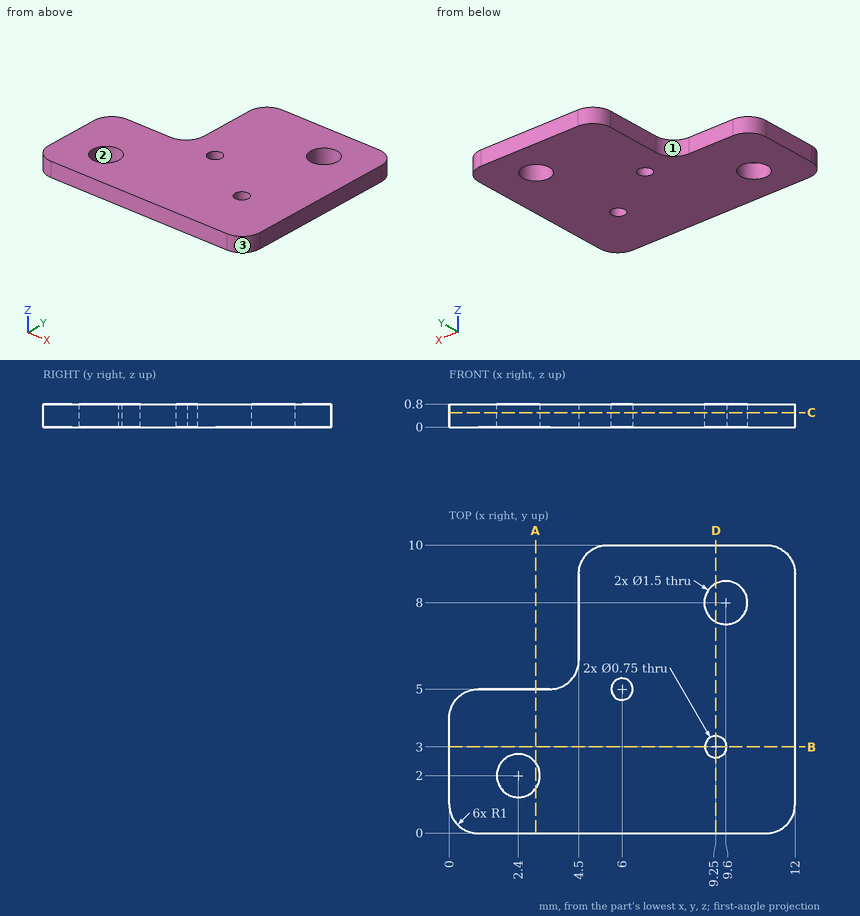
Geometry: see drawing. Coordinates: mm, zero at the bounding-box minimum. Round coordinates to 2 decimals unless told otherwise and drop trailing zeros. Loops run counter-clockwise (first coordinate to the right, second up) from the corner with the lowest first, then second, coordinate; pieces in that order, holes last. Notation, with made-up numbers: M 86.5,16 L 106.5,16 A33 ccw 106.5,55 Z; hole C 15.5,5 d8. An arc over 180 degrees is marked long. Use a Markdown table: item, result. Add a question column.
1. Contact query for a flat-ended pin moving along its axis: pin 1 (1.2 mm diameter, centred on x = 2.4, y = 2, fed in from -Z). Output: stop coordinate, or through.
2. Cut plane D-D, the plane x = 9.25. Output: boundary loops of the cut face in (y, z) (3 decimals).
3. Cut plane A-A, the plane x = 3. Output: boundary loops of the cut face in (y, z), and give its area (3 significant figures).
4. Pull-direction query (Y, two-part tool) for the marked faces 1, 2 and 3; classes: +Y half, -Y half, draft (parallel to the pull), parting line (faces both ways), or undercut.
5. Cut plane C-C, the plane z = 0.5. Output: boundary loops of the cut face in (x, y) (3 decimals), and give its area (3 significant figures).
6. Cut plane B-B, the plane y = 3. Output: boundary loops of the cut face in (x, z) (3 decimals).
7. Ray query, line 1 along Y through (x, z) = (9.25, 0.55) (3 decimals); line 2 along Y through (x, z) = (6, 0.45) (3 decimals); line 3 along X through (y, z) = (9, 0.1). Return the intervals inside material, ascending. Write a range as [from, to].
Solution:
| question | item | result |
|---|---|---|
| 1 | pin 1 | passes through |
| 2 | outline | M 0,0 L 2.625,0 L 2.625,0.8 L 0,0.8 Z; M 3.375,0 L 7.337,0 L 7.337,0.8 L 3.375,0.8 Z; M 8.663,0 L 10,0 L 10,0.8 L 8.663,0.8 Z |
| 3 | outline | M 0,0 L 1.55,0 L 1.55,0.8 L 0,0.8 Z; M 2.45,0 L 5,0 L 5,0.8 L 2.45,0.8 Z |
| 3 | area | 3.28 mm2 |
| 4 | face 1 | +Y half |
| 4 | face 2 | undercut |
| 4 | face 3 | -Y half |
| 5 | outline | M 0,1 A1 ccw 1,0 L 11,0 A1 ccw 12,1 L 12,9 A1 ccw 11,10 L 5.5,10 A1 ccw 4.5,9 L 4.5,6 A1 cw 3.5,5 L 1,5 A1 ccw 0,4 Z; hole C 2.4,2 d1.5; hole C 6,5 d0.75; hole C 9.6,8 d1.5; hole C 9.25,3 d0.75 |
| 5 | area | 92.2 mm2 |
| 6 | outline | M 0,0 L 8.875,0 L 8.875,0.8 L 0,0.8 Z; M 9.625,0 L 12,0 L 12,0.8 L 9.625,0.8 Z |
| 7 | line 1 | y = [0, 2.625], [3.375, 7.337], [8.663, 10] |
| 7 | line 2 | y = [0, 4.625], [5.375, 10] |
| 7 | line 3 | x = [4.5, 12] |
